Source: CAD feature listing. Evaluate the final solid. Frame: model axes, mm. Round coordinates to 2 decimals unless told otherwise and drop trailing zeros. Loops run counter-clockwise (first coordinate to the right, second up) from the corner with the lowest first, then second, coordinate; pieces in that order, holes last. Notation, with made-up numbers: (-38.75, 46.5) -> (-22.75, 46.5) arc R3 ccw to (-22.75, 51.5) -> close; hole circle Ø4 at (1.5, -36). An arc over 180 degrees is marked (long way). Put each result on its own line as item: value. Start each with the question number.
1. Cut plane A-A (z = 1.45). Return the cut outline in (x, y), then the cut area to 3 significant figures.
2. Cut plane C-C (x = -3.5). Return the cut outline in (y, z), then the cut area to 3 significant figures.
3. Contact query for flat-ended pins moving along their axis: pin 1 (1 mm diameter, centred on x = 1, z = 2, fed in from -Y); pin 2 (1 mm diameter, centred on y = -12, z = 2, fed in from -X). Output: stop coordinate, or through.
4. Material intervals for L1, parallel to Y at x = -3, z = 2.4; L2, parallel to X at y = -20, z = 2.85; L3, parallel to Y at x = 6, z = 0.2, sorted ascending.
5. Cut plane B-B (y = -26). Return the cut outline in (x, z), then the cut area to 3 significant figures.
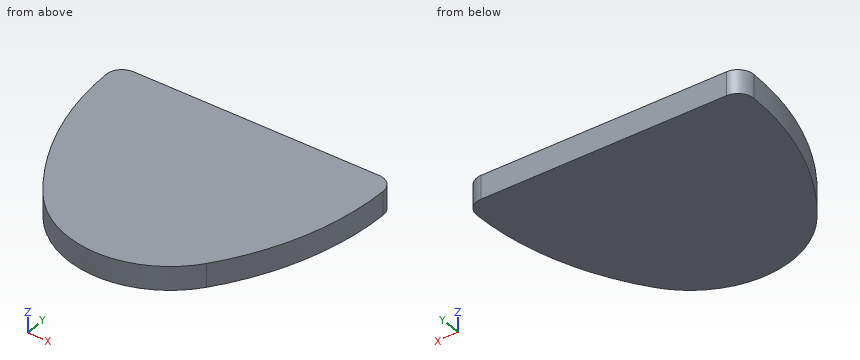
```python
from build123d import *

# Parameters (mm, degrees)
F1_DEPTH = 3


with BuildPart() as f1:
    # F0 (on Top) → F1 (new body)
    with BuildSketch(Plane.XY):
        with BuildLine():
            Line((0, 0), (-15.5, 0))
            ThreePointArc((-15.5, 0), (-16.921363, -0.592973), (-17.499897, -2.020274))
            ThreePointArc((-17.499897, -2.020274), (-15.60578, -13.028563), (-10.339907, -22.879487))
            ThreePointArc((-10.339907, -22.879487), (0, -28), (10.339907, -22.879487))
            ThreePointArc((10.339907, -22.879487), (15.60578, -13.028563), (17.499897, -2.020274))
            ThreePointArc((17.499897, -2.020274), (16.921363, -0.592973), (15.5, 0))
            Line((15.5, 0), (0, 0))
        make_face()
    extrude(amount=F1_DEPTH)


solid = f1.part
```
Solution:
1. outline: (-17.5, -2.02) arc R35 ccw to (-10.34, -22.88) arc R13 ccw to (10.34, -22.88) arc R35 ccw to (17.5, -2.02) arc R2 ccw to (15.5, 0) -> (-15.5, 0) arc R2 ccw to start
1. area: 776 mm^2
2. outline: (-27.52, 0) -> (0, 0) -> (0, 3) -> (-27.52, 3) -> close
2. area: 82.6 mm^2
3. pin 1: stops at y = -27.99
3. pin 2: stops at x = -16.09
4. L1: y = -27.65 to 0
4. L2: x = -12.32 to 12.32
4. L3: y = -26.53 to 0
5. outline: (-6.93, 0) -> (6.93, 0) -> (6.93, 3) -> (-6.93, 3) -> close
5. area: 41.6 mm^2
